Autodesk Inventor part; units mm, degrees
ref_plane "YZ Plane" through (0, 0, 0) normal (1, 0, 0) x (0, 1, 0)
ref_plane "XZ Plane" through (0, 0, 0) normal (0, 1, 0) x (-1, 0, 0)
ref_plane "XY Plane" through (0, 0, 0) normal (0, 0, 1) x (1, 0, 0)
sketch "Esboço1" plane through (0, 0, 0) normal (0, 0, 1) x (1, 0, 0)
  circle A0 centre (0, 0) radius 5
  dimension "d0" = 10
extrude "Extrusão1" add sketch "Esboço1" along normal mid plane 80
sketch "Esboço2" plane through (0, 0, 0) normal (1, 0, 0) x (0, 1, 0)
  line L0 (5, -40) -> (5, 40)
  line L1 (5, 36.8) -> (4, 36.8)
  line L2 (4, 36.8) -> (4, 35.8)
  line L3 (4, 35.8) -> (5, 35.8)
  line L4 (5, 35.8) -> (5, 36.8)
  line L5 (4, -35.8) -> (5, -35.8)
  line L6 (5, -35.8) -> (5, -36.8)
  line L7 (5, -36.8) -> (4, -36.8)
  line L8 (4, -36.8) -> (4, -35.8)
  line L9 (5, 40) -> (-5, 40)
  line L10 (-5, -40) -> (5, -40)
  line L11 (0, -56) -> (0, 56)
  point P0 (0, 0)
  dimension "d3" = 4.2
  dimension "d4" = 1
  dimension "d5" = 4
  dimension "d6" = 1
  dimension "d7" = 4.2
revolve "Revolução1" cut sketch "Esboço2" angle 360 about axis through (0, 0, -10) along (0, 0, 1) contours L7 L8 L5 L0 | L3 L2 L1 L0
chamfer "Chanfro1" distance 0.5 angle 45 2 edges at (-5, 0, 40) (-5, 0, -40)
Build history of the part. All positions in model axes, mm. Coordinates: 2 decimals unless noted, no trailing zeros. Order: outer loops, then holes, each group sorted by start corner. A loop starts at its lowest first (then second) coordinate and runs counter-clockwise, first axis right, second up. Notation, with made-up numbers: M 84.5,50 L 101.5,50 A22 ccw 101.5,80 Z; hole C 41,-22 d8. An arc over 180 degrees is marked long. One line per question, with ' | ' between items. Start each with the question number.
1. Wall check: line 1 along Z through (x, y) = (0, -4.25); line 2 along Z through (x, y) = (0.75, -4.5); line 3 along Y through (x, z) = (-3, 12.5). Give the ranges that are in metal, low to high. Write a range as [from, to].
2. Mould opens along Z. For faces 1 (the face through (-3.905, -0.867, 36.293)), 2 (the face through (3.905, -0.867, -36.293)), 3 (the face through (-1.08, 4.88, -0.5)), 4 (the face through (0, 0, 40)) say: +Z half, -Z half, draft (parallel to the pull), parting line (faces both ways), or undercut.
3. Flat gauge pin, fed straight in: P1, Ø1, axis at y = -1, z = -15.5, coming from the -X side. Where does the tip first touch, or does it go through?
4. Cut at A-A (z = -28.5). Write the cut outline in (x, y), plus the area to 3 significant figures.
The answers:
1) line 1: z = [-40, -36.8], [-35.8, 35.8], [36.8, 40] | line 2: z = [-39.94, -36.8], [-35.8, 35.8], [36.8, 39.94] | line 3: y = [-4, 4]
2) face 1: undercut | face 2: undercut | face 3: draft | face 4: +Z half
3) P1: stops at x = -4.97
4) outline: C 0,0 d10 | area: 78.5 mm2
